Here's how the part is built. I have some questions about the finished solid (model axes, mm). Give positions to 0.01 mm unless a question says otherwise; leave off trailing zeros. Loops run counter-clockwise (first coordinate to the right, second up) from the corner with the lowest first, then second, coordinate; pieces in that order, holes last. Notation, with made-up numbers: (2.25, 12) - (32.25, 12) arc R33 cw to (32.25, 49) - close; hole circle Ø9 at (13, -34). An arc over 180 degrees is marked (long way). Use one line per item in the form item = value.
from build123d import *

# Parameters (mm, degrees)
SKETCH1_R                 = 0.9906
SKETCH1_R_2               = 1.6
SKETCH1_R_3               = 3.5
BOSS_EXTRUDE2_DEPTH       = 3.175
F_2_CLEARANCE_HOLE1_D     = 2.4384
F_2_CLEARANCE_HOLE1_DEPTH = 3.302
F_2_CLEARANCE_HOLE1_TIP   = 0.732569267


with BuildPart() as part:
    # Sketch1 → Boss-Extrude2 (new body)
    with BuildSketch(Plane.XY):
        with BuildLine():
            Line((0, 0), (37, 0))
            Line((37, 0), (37, 6.50213794))
            ThreePointArc((37, 6.50213794), (30.666699296, 13), (37, 19.49786206))
            Line((37, 19.49786206), (37, 30))
            Line((37, 30), (0, 30))
            Line((0, 30), (0, 0))
        make_face()
        with Locations((25.169778966, 20.933400182)):
            Circle(SKETCH1_R, mode=Mode.SUBTRACT)
        with Locations((16, 24.5)):
            Circle(SKETCH1_R_2, mode=Mode.SUBTRACT)
        with Locations((24, 15)):
            Circle(SKETCH1_R_2, mode=Mode.SUBTRACT)
        with Locations(Location((16, 5.5, 0), (0, 0, 180))):
            Circle(SKETCH1_R_2, mode=Mode.SUBTRACT)
        with Locations(Location((8, 15, 0), (0, 0, 180))):
            Circle(SKETCH1_R_2, mode=Mode.SUBTRACT)
        with Locations((16, 15)):
            Circle(SKETCH1_R_3, mode=Mode.SUBTRACT)
    extrude(amount=BOSS_EXTRUDE2_DEPTH)

    # #2 Clearance Hole1
    with Locations(Plane.XY.offset(3.175)):
        with Locations((3, 27), (3, 3), (34, 3), (34, 27)):
            Hole(F_2_CLEARANCE_HOLE1_D / 2, depth=F_2_CLEARANCE_HOLE1_DEPTH)
            with Locations((0, 0, -(F_2_CLEARANCE_HOLE1_DEPTH + F_2_CLEARANCE_HOLE1_TIP / 2))):  # 118° drill point
                Cone(0, F_2_CLEARANCE_HOLE1_D / 2, F_2_CLEARANCE_HOLE1_TIP, mode=Mode.SUBTRACT)


solid = part.part
(1) Thinking about a two-plate mould opening in Y: for faces 1 (the cylindrical face through (23.792, 16.586, 1.565)), 2 (the cylindrical face through (17.6, 5.43, 1.57)), 3 (the flat face through (18, 0, 2)), 4 (the flat face through (0, 15, 2)), which applies, pulls with the +Y half, pulls with the -Y half, needs draft (parallel to the pull), parting line crosses it, or undercut?
Geometry says:
face_1 = undercut
face_2 = undercut
face_3 = pulls with the -Y half
face_4 = needs draft
(2) If we section it at B-B (x = 3): List the corners of the cut face in (y, z) for me (3 decimals), plus the area to 3 significant figures.
Geometry says:
outline = (0, 0) - (1.781, 0) - (1.781, 3.175) - (0, 3.175) - close; (4.219, 0) - (25.781, 0) - (25.781, 3.175) - (4.219, 3.175) - close; (28.219, 0) - (30, 0) - (30, 3.175) - (28.219, 3.175) - close
area = 79.8 mm²
(3) For P1, Ø3, axis at x = 34, y = 27, coming from the -Z side, with a flat end and sliding along its axis, tell me the tip position at first contact or that it passes through.
Geometry says:
P1 = 0
(4) If we section it at D-D (y = 17): List the corners of the cut face in (x, z) for me (3 decimals).
Geometry says:
outline = (0, 0) - (13.128, 0) - (13.128, 3.175) - (0, 3.175) - close; (18.872, 0) - (32.043, 0) - (32.043, 3.175) - (18.872, 3.175) - close
(5) If I drill on probe 1 along Y at (x, z) = (34, 2.55); probe 2 along X at (y, z) = (2.75, 1.1); probe 3 along X at (y, z) = (13.25, 2.05), over which ranges is the centre line in solid material (lowest first)?
Geometry says:
probe_1 = 0 to 1.78, 4.22 to 7.32, 18.68 to 25.78, 28.22 to 30
probe_2 = 0 to 1.81, 4.19 to 32.81, 35.19 to 37
probe_3 = 0 to 12.97, 19.03 to 30.67
(6) If we section it at A-A (y = 27): List the corners of the cut face in (x, z) for me (3 decimals).
Geometry says:
outline = (0, 0) - (1.781, 0) - (1.781, 3.175) - (0, 3.175) - close; (4.219, 0) - (32.781, 0) - (32.781, 3.175) - (4.219, 3.175) - close; (35.219, 0) - (37, 0) - (37, 3.175) - (35.219, 3.175) - close
(7) If we section it at C-C (x = 16): List the corners of the cut face in (y, z) for me (3 decimals).
Geometry says:
outline = (0, 0) - (3.9, 0) - (3.9, 3.175) - (0, 3.175) - close; (7.1, 0) - (11.5, 0) - (11.5, 3.175) - (7.1, 3.175) - close; (18.5, 0) - (22.9, 0) - (22.9, 3.175) - (18.5, 3.175) - close; (26.1, 0) - (30, 0) - (30, 3.175) - (26.1, 3.175) - close
